For this review, take the finished solid that the model builds, in its own axes (mm). A direction names the side the tool comes from. Round coordinates to 2 decimals unless told otherwise and drop trailing zeros. Order: outer loops, then holes, each group sorted by start corner. A loop starts at its lowest first (then second) coordinate and runs counter-clockwise, first axis right, second up. Notation, with made-up numbers: M 1.25,-1.75 L 26.25,-1.75 A31 cw 26.25,26.25 Z; hole C -3,13 d7. An arc over 180 degrees is marked long. Answer in a Markdown table with one row per item. Add a question column.
```python
from build123d import *

# Parameters (mm, degrees)
F0_W     = 76.2
F0_H     = 63.5
F1_DEPTH = 76.2
F2_T     = -2.54
F3_W     = 27.94
F3_H     = 27.94
F4_DEPTH = 16.256
F5_W     = 40.64
F5_H     = 21.59
F6_DEPTH = 100.076
F7_R     = 3.81
F8_DEPTH = 99.822


with BuildPart() as f1:
    # F0 (on Front) → F1 (new body)
    with BuildSketch(Plane.XZ):
        with Locations((-22.039793, 29.765201)):
            Rectangle(F0_W, F0_H)
        Polygon((38.920207, -1.984799), (16.060207, 61.515201), (16.060207, -1.984799), align=None)
    extrude(amount=F1_DEPTH)

    # F2
    f2_openings = [f1.faces().sort_by_distance(p)[0] for p in [
        (-22.039793, -38.1, 61.515201),
    ]]
    offset(amount=F2_T, openings=f2_openings)

    # F3 (on face) → F4 (cut)
    with BuildSketch(Plane(origin=(0, 0, -1.984799), x_dir=(1, 0, 0), z_dir=(0, 0, -1))):
        with Locations((14.790207, 38.1)):
            Rectangle(F3_W, F3_H)
    extrude(amount=-F4_DEPTH, mode=Mode.SUBTRACT)

    # F5 (on face) → F6 (cut)
    with BuildSketch(Plane.XZ.offset(76.2)):
        with Locations((-36.9158, 10.795)):
            Rectangle(F5_W, F5_H)
    extrude(amount=-F6_DEPTH, mode=Mode.SUBTRACT)

    # F7 (on face) → F8 (cut)
    with BuildSketch(Plane.XZ.offset(76.2)):
        with Locations((22.432121, 8.792778)):
            Circle(F7_R)
    extrude(amount=-F8_DEPTH, mode=Mode.SUBTRACT)


solid = f1.part
```
1. To check wall thickness, follow probe 1 along Y at (x, z) = (-18.5, 32.5); probe 2 along Z at (x, y) = (-31, -21); probe 3 along X at (y, z) = (-60, 58). State the ranges of each line that lie inside material, in increasing order. Write a range as [from, to].
2. Consider section C-C on x = -35. Write out the cut boundary in (y, z), plus the area to 3 significant figures.
3. Consider section D-D on z = 10.5. Write out the cut boundary in (x, y).
4. For faces 1 (the flat face through (15, -24.13, -1)), 2 (the flat face through (-12, -2.54, 31)), 3 (the flat face through (-57.6, -38, 31)), list the 3-axis set-ups (+Z, -Z, +X, -X, +Y, -Y) from which the entire face can be reached by the end or side of a thin tool; tool diameter is ignored.
5. Clearance check with flat-ended pins moving along their axes: pin 1 Ø23.5 at (y, z) = (-33.5, 13.5) entering from +X; pin 2 Ø2 at (y, z) = (-45, -0.5) entering from +X; pin 3 Ø12 at (y, z) = (-44, 23.5) entering from +X; pin 4 Ø7 at (x, z) = (22.43, 8.79) entering from +Y. State where each tip first meets the part, or that it passes through.
6. Consider section A-A on x = 3.5. Write out the cut boundary in (y, z).
7. Consider section B-B on y = -45. Write out the cut boundary in (x, z).
8. The part is to be moulded in two halves that separate along Z. For faces 4 (the flat face through (-25, -75, 61.515)), 5 (the flat face through (-11, 0, 30)), 6 (the flat face through (-11, -38, -1.985)), 7 (the flat face through (-37, -1, 21.59)), say which applies: pulls with the +Z half, pulls with the -Z half, needs draft (parallel to the pull), parting line crosses it, or undercut.
Solved:
| question | item | result |
|---|---|---|
| 1 | probe 1 | y = [-76.2, -73.66], [-2.54, 0] |
| 1 | probe 2 | z = [-1.98, 0] |
| 1 | probe 3 | x = [-60.14, -57.6], [14.63, 17.33] |
| 2 | outline | M -76.2,-1.98 L 0,-1.98 L 0,0 L -76.2,0 Z; M -76.2,21.59 L -73.66,21.59 L -73.66,61.52 L -76.2,61.52 Z; M -2.54,21.59 L 0,21.59 L 0,61.52 L -2.54,61.52 Z |
| 2 | area | 354 mm^2 |
| 3 | outline | M -60.14,-76.2 L -57.24,-76.2 L -57.24,-73.66 L -57.6,-73.66 L -57.6,-2.54 L -57.24,-2.54 L -57.24,0 L -60.14,0 Z; M -16.6,-76.2 L 19.03,-76.2 L 19.03,-73.66 L -16.6,-73.66 Z; M -16.6,-2.54 L 19.03,-2.54 L 19.03,0 L -16.6,0 Z; M 25.84,-76.2 L 34.43,-76.2 L 34.43,0 L 25.84,0 L 25.84,-2.54 L 31.73,-2.54 L 31.73,-73.66 L 25.84,-73.66 Z |
| 4 | face 1 | -Z |
| 4 | face 2 | none |
| 4 | face 3 | +Z |
| 5 | pin 1 | stops at x = 37.58 |
| 5 | pin 2 | stops at x = 38.75 |
| 5 | pin 3 | stops at x = 31.91 |
| 5 | pin 4 | passes through |
| 6 | outline | M -76.2,-1.98 L -52.07,-1.98 L -52.07,0.56 L -73.66,0.56 L -73.66,61.52 L -76.2,61.52 Z; M -24.13,-1.98 L 0,-1.98 L 0,61.52 L -2.54,61.52 L -2.54,0.56 L -24.13,0.56 Z |
| 7 | outline | M -60.14,-1.98 L 0.82,-1.98 L 0.82,0.56 L -16.6,0.56 L -16.6,0 L -57.24,0 L -57.24,0.56 L -57.6,0.56 L -57.6,61.52 L -60.14,61.52 Z; M 13.36,61.52 L 35.31,0.56 L 28.76,0.56 L 28.76,-1.98 L 38.92,-1.98 L 16.06,61.52 Z |
| 8 | face 4 | pulls with the +Z half |
| 8 | face 5 | needs draft |
| 8 | face 6 | pulls with the -Z half |
| 8 | face 7 | undercut |
